Autodesk Inventor part; units mm, degrees
ref_plane "YZ Plane" through (0, 0, 0) normal (1, 0, 0) x (0, 1, 0)
ref_plane "XZ Plane" through (0, 0, 0) normal (0, 1, 0) x (-1, 0, 0)
ref_plane "XY Plane" through (0, 0, 0) normal (0, 0, 1) x (1, 0, 0)
sketch "Sketch1" plane through (0, 0, 0) normal (0, 1, 0) x (-1, 0, 0)
  line L0 (51.9615, 0) -> (25.9808, -45)
  line L1 (25.9808, -45) -> (-25.9808, -45)
  line L2 (-25.9808, -45) -> (-51.9615, 0)
  line L3 (-51.9615, 0) -> (-25.9808, 45)
  line L4 (-25.9808, 45) -> (25.9808, 45)
  line L5 (25.9808, 45) -> (51.9615, 0)
  point P0 (0, 0)
  point P1 (0, 0)
  dimension "d1" = 45
  dimension "d2" = 45
extrude "Extrusion1" add sketch "Sketch1" along normal blind 5
sketch "Sketch2" plane through (0, 5, 0) normal (0, 1, 0) x (1, 0, 0)
  line L0 (-25.9808, 45) -> (-51.9615, 0)
  line L1 (-38.9711, 22.5) -> (-47.9711, 6.9115)
  line L2 (-38.9711, 22.5) -> (-29.9711, 38.0885)
  line L3 (-47.9711, 6.9115) -> (-40.1769, 2.4115)
  line L4 (-38.226, 8.7907) -> (-44.726, -2.4676)
  line L5 (-44.726, -2.4676) -> (-42.1279, -3.9676)
  line L6 (-42.1279, -3.9676) -> (-35.6279, 7.2907)
  line L7 (-35.6279, 7.2907) -> (-38.226, 8.7907)
  line L8 (-38.226, 8.7907) -> (-42.1279, -3.9676) construction
  line L9 (-44.726, -2.4676) -> (-35.6279, 7.2907) construction
  line L10 (-38.226, 8.7907) -> (-25.226, 8.7907) construction
  line L11 (-29.9711, 38.0885) -> (-22.1769, 33.5885)
  line L12 (-17.6279, 38.4676) -> (-24.1279, 27.2093)
  line L13 (-24.1279, 27.2093) -> (-26.726, 28.7093)
  line L14 (-26.726, 28.7093) -> (-20.226, 39.9676)
  line L15 (-20.226, 39.9676) -> (-17.6279, 38.4676)
  line L16 (-17.6279, 38.4676) -> (-26.726, 28.7093) construction
  line L17 (-24.1279, 27.2093) -> (-20.226, 39.9676) construction
  circle A0 centre (0, 0) radius 0.5
  dimension "d5" = 18
  dimension "d6" = 18
  dimension "d7" = 9
  dimension "d8" = 90
  dimension "d9" = 13
  dimension "d10" = 120
  dimension "d11" = 3
  dimension "d12" = 9
  dimension "d13" = 13
  dimension "d14" = 3
  dimension "d15" = 90
  dimension "d16" = 1
extrude "Extrusion2" cut sketch "Sketch2" against normal blind 5
pattern_circular "Circular Pattern1" count 3 over 360 about axis through (0, 5, 0) along (0, -1, 0) of "Extrusion2"
fillet "Fillet1" radius 5 6 edges at (38.9711, 5, 22.5) (38.9711, 5, -22.5) (0, 5, -45) (-38.9711, 5, -22.5) (-38.9711, 5, 22.5) (0, 5, 45)
properties part number "Bot_"
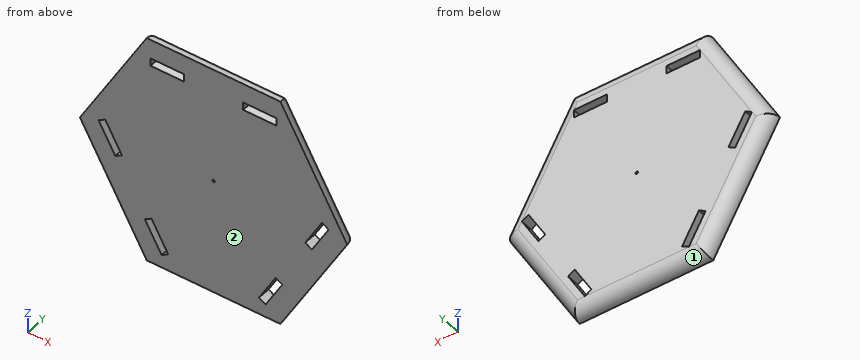
CAD build for the part. Positions are in the model's coordinates, mm. Face numbers are marked on the shaded views. Coordinates: 2 decimals unless noted, no trailing zeros. Use CSV: the item, a comma, the result in double quotes. Start each with the question number.
Item 1: Wall check: probe 1 along X at (y, z) = (3.2, 0); probe 2 along X at (y, z) = (2.2, 0); probe 3 along X at (y, z) = (2.95, -4). Give the ranges that are in metal, low to high.
Item 2: Band-saw the part on A-A, the plane y = 3. Give the number of separate pieces and of enclosed holes in the cut face, plus the area to 3 significant figures.
Item 3: Drop flat-ended pins along their axis: P1, Ø1.5, axis at x = 17.5, y = 3.5, coming from the +Z side; P2, Ø1.5, axis at y = 3.5, z = 3.5, coming from the -X side; P3, Ø0.9, axis at y = 3, z = 36.5, coming from the +X side. Give the stop position or say it passes through.
Item 4: Two-plate mould, pull along Y, no slides. Class the marked faces 1 and 2: +Y half, -Y half, draft (parallel to the pull), parting line (faces both ways), or undercut.
Response values:
1,probe 1,"x = -50.62 to -43.3, -39.84 to -0.5, 0.5 to 39.84, 43.3 to 50.62"
1,probe 2,"x = -51.37 to -43.3, -39.84 to -0.5, 0.5 to 39.84, 43.3 to 51.37"
1,probe 3,"x = -48.54 to -40.99, -37.53 to 37.53, 40.99 to 48.54"
2,separate pieces,"1"
2,enclosed holes,"7"
2,area,"6,470 mm2"
3,P1,"stops at z = 44.18"
3,P2,"stops at x = -49.13"
3,P3,"stops at x = 30.17"
4,face 1,"+Y half"
4,face 2,"-Y half"
